Work out the finished part from the listing and answer in its coordinate system (mm). A direction names the side the tool comes from. Round coordinates to 2 decimals unless told otherwise and drop trailing zeros. Order: outer loops, then holes, each group sorted by start corner. A loop starts at its lowest first (then second) coordinate and runs counter-clockwise, first axis right, second up. Notation, with made-up numbers: (39, 29) -> (60, 29) arc R23 cw to (60, 58) -> close; hole circle Ø7 at (29.5, 17). An arc over 180 degrees is marked (long way). Use a Markdown table: item, result. Add a question column.
Item 1: Find the intervals of material crossed by L1, parallel to X at y = -52, z = 1.5; L2, parallel to Y at x = -55, z = 4.5 (3 decimals); L3, parallel to Z at x = 2.5, y = 0 (3 decimals), in increasing order. Write a range as [from, to].
Item 2: A cutting plane is placed at D-D, the plane x = -25. Determine the outline of the cut face in (y, z) (3 decimals), plus the area to 3 significant figures.
Item 3: A cutting plane is placed at C-C, the plane y = -50.5. Determine the outline of the cut face in (x, z).
Item 4: For a pull along X with two mould halves and no side action, classify faces 5 (the flat face through (-51, 38.1, 3)), 6 (the flat face through (-1, 1, 0)), 7 (the cylindrical face through (-72.38, 72.58, 3.13)) as +X half, -X half, draft (parallel to the pull), parting line (faces both ways), or undercut.
Item 5: A cutting plane is placed at B-B, the plane z = 3.5. Determine the outline of the cut face in (x, y) (3 decimals), plus the area to 3 significant figures.
Item 6: A cutting plane is placed at A-A, the plane y = 0. Determine the outline of the cut face in (x, z) (3 decimals), plus the area to 3 significant figures.
Item 7: A tool of negligible diameter and unlimited length cuts with its end or side. For faces 1 (the flat face through (51, -41.275, 3)), 2 (the flat face through (-31.75, -1, 25)), 3 (the flat face through (31.75, -1, 25)), 4 (the flat face through (0, 63.5, 19)), from which of +Z, -Z, +X, -X, +Y, -Y can it reach the whole face along a straight path? Write none if from no direction.
Item 8: Flat-ended cylindrical pins translate along their axes: P1, Ø4, axis at y = -54, z = 15.5, coming from the -X side; P2, Ø14.5, axis at y = 0, z = 15.875, coming from the +X side; P3, Ø3, axis at x = 26.5, z = 21.5, coming from the +Y side. Find the tip coordinate at first contact, or state that the pin passes through.
from build123d import *

# Parameters (mm, degrees)
F2_DEPTH = 6.35
F3_W     = 63.5
F3_H     = 127
F4_DEPTH = 25.4
F5_R     = 6.35
F6_DEPTH = 63.5
F7_W     = 12.7
F7_H     = 25.4
F8_DEPTH = 6.35


# Not quite as in the source:
# - the program builds the solid bodies; features that only make, move or delete a surface that nothing else refers to are left out


with BuildPart() as f2:
    # F0 (on Top) → F2 (new body)
    with BuildSketch(Plane.XY):
        with BuildLine():
            Line((63.5, 76.2), (-63.5, 76.2))
            ThreePointArc((-63.5, 76.2), (-72.4802561211, 72.4802561211), (-76.2, 63.5))
            Line((-76.2, 63.5), (-76.2, -63.5))
            ThreePointArc((-76.2, -63.5), (-72.4802561211, -72.4802561211), (-63.5, -76.2))
            Line((-63.5, -76.2), (63.5, -76.2))
            ThreePointArc((63.5, -76.2), (72.4802561211, -72.4802561211), (76.2, -63.5))
            Line((76.2, -63.5), (76.2, 63.5))
            ThreePointArc((76.2, 63.5), (72.4802561211, 72.4802561211), (63.5, 76.2))
        make_face()
        with BuildLine():
            ThreePointArc((-69.85, 57.15), (-66.1302561211, 66.1302561211), (-57.15, 69.85))
            Line((-57.15, 69.85), (-1.846e-07, 69.85))
            Line((-1.846e-07, 69.85), (57.15, 69.85))
            ThreePointArc((57.15, 69.85), (66.1302561211, 66.1302561211), (69.85, 57.15))
            Line((69.85, 57.15), (69.85, 0))
            Line((69.85, 0), (69.85, -57.15))
            ThreePointArc((69.85, -57.15), (66.1302561211, -66.1302561211), (57.15, -69.85))
            Line((57.15, -69.85), (0, -69.85))
            Line((0, -69.85), (-57.15, -69.85))
            ThreePointArc((-57.15, -69.85), (-66.1302561211, -66.1302561211), (-69.85, -57.15))
            Line((-69.85, -57.15), (-69.85, -1.807e-07))
            Line((-69.85, -1.807e-07), (-69.85, 57.15))
        make_face(mode=Mode.SUBTRACT)
        with BuildLine():
            ThreePointArc((69.85, 0), (49.3914086006, 49.3914087312), (-1.846e-07, 69.85))
            ThreePointArc((-1.846e-07, 69.85), (-49.3914087951, 49.3914085367), (-69.85, -1.807e-07))
            ThreePointArc((-69.85, -1.807e-07), (-49.391408602, -49.3914087298), (0, -69.85))
            ThreePointArc((0, -69.85), (49.3914086659, -49.3914086659), (69.85, 0))
        make_face()
        with BuildLine():
            Line((57.15, 69.85), (-1.846e-07, 69.85))
            ThreePointArc((-1.846e-07, 69.85), (49.3914086006, 49.3914087312), (69.85, 0))
            Line((69.85, 0), (69.85, 57.15))
            ThreePointArc((69.85, 57.15), (66.1302561211, 66.1302561211), (57.15, 69.85))
        make_face()
        with BuildLine():
            Line((-1.846e-07, 69.85), (-57.15, 69.85))
            ThreePointArc((-57.15, 69.85), (-66.1302561211, 66.1302561211), (-69.85, 57.15))
            Line((-69.85, 57.15), (-69.85, -1.807e-07))
            ThreePointArc((-69.85, -1.807e-07), (-49.3914087951, 49.3914085367), (-1.846e-07, 69.85))
        make_face()
        with BuildLine():
            Line((69.85, -57.15), (69.85, 0))
            ThreePointArc((69.85, 0), (49.3914086659, -49.3914086659), (0, -69.85))
            Line((0, -69.85), (57.15, -69.85))
            ThreePointArc((57.15, -69.85), (66.1302561211, -66.1302561211), (69.85, -57.15))
        make_face()
        with BuildLine():
            ThreePointArc((0, -69.85), (-49.391408602, -49.3914087298), (-69.85, -1.807e-07))
            Line((-69.85, -1.807e-07), (-69.85, -57.15))
            ThreePointArc((-69.85, -57.15), (-66.1302561211, -66.1302561211), (-57.15, -69.85))
            Line((-57.15, -69.85), (0, -69.85))
        make_face()
    extrude(amount=F2_DEPTH)

    # F3 (on face) → F4 (join)
    with BuildSketch(Plane.XY.offset(6.35)):
        Rectangle(F3_W, F3_H)
    extrude(amount=F4_DEPTH)

    # F5 (on face) → F6 (cut)
    with BuildSketch(Plane.YZ.offset(31.75)):
        with Locations((0, 15.875)):
            Circle(F5_R)
    extrude(amount=-F6_DEPTH, mode=Mode.SUBTRACT)

    # F7 (on face) → F8 (cut)
    with BuildSketch(Plane.XY.offset(6.35)):
        with Locations((50.8, 25.4)):
            Rectangle(F7_W, F7_H)
        with Locations((-50.8, 25.4)):
            Rectangle(F7_W, F7_H)
        with Locations((-50.8, -53.975)):
            Rectangle(F7_W, F7_H)
        with Locations((50.8, -53.975)):
            Rectangle(F7_W, F7_H)
    extrude(amount=-F8_DEPTH, mode=Mode.SUBTRACT)


solid = f2.part
Reported:
| question | item | result |
|---|---|---|
| 1 | L1 | [-76.2, -57.15], [-44.45, 44.45], [57.15, 76.2] |
| 1 | L2 | [-76.2, -66.675], [-41.275, 12.7], [38.1, 76.2] |
| 1 | L3 | [0, 9.525], [22.225, 31.75] |
| 2 | outline | (-76.2, 0) -> (76.2, 0) -> (76.2, 6.35) -> (63.5, 6.35) -> (63.5, 31.75) -> (-63.5, 31.75) -> (-63.5, 6.35) -> (-76.2, 6.35) -> close; hole circle Ø12.7 at (0, 15.875) |
| 2 | area | 4,070 mm² |
| 3 | outline | (-76.2, 0) -> (-57.15, 0) -> (-57.15, 6.35) -> (-76.2, 6.35) -> close; (-44.45, 0) -> (44.45, 0) -> (44.45, 6.35) -> (31.75, 6.35) -> (31.75, 31.75) -> (-31.75, 31.75) -> (-31.75, 6.35) -> (-44.45, 6.35) -> close; (57.15, 0) -> (76.2, 0) -> (76.2, 6.35) -> (57.15, 6.35) -> close |
| 4 | face 5 | undercut |
| 4 | face 6 | draft |
| 4 | face 7 | -X half |
| 5 | outline | (-76.2, -63.5) arc R12.7 ccw to (-63.5, -76.2) -> (63.5, -76.2) arc R12.7 ccw to (76.2, -63.5) -> (76.2, 63.5) arc R12.7 ccw to (63.5, 76.2) -> (-63.5, 76.2) arc R12.7 ccw to (-76.2, 63.5) -> close; hole (-57.15, -66.675) -> (-44.45, -66.675) -> (-44.45, -41.275) -> (-57.15, -41.275) -> close; hole (-57.15, 12.7) -> (-44.45, 12.7) -> (-44.45, 38.1) -> (-57.15, 38.1) -> close; hole (44.45, -66.675) -> (57.15, -66.675) -> (57.15, -41.275) -> (44.45, -41.275) -> close; hole (44.45, 12.7) -> (57.15, 12.7) -> (57.15, 38.1) -> (44.45, 38.1) -> close |
| 5 | area | 21,800 mm² |
| 6 | outline | (-76.2, 0) -> (76.2, 0) -> (76.2, 6.35) -> (31.75, 6.35) -> (31.75, 9.525) -> (-31.75, 9.525) -> (-31.75, 6.35) -> (-76.2, 6.35) -> close; (-31.75, 22.225) -> (31.75, 22.225) -> (31.75, 31.75) -> (-31.75, 31.75) -> close |
| 6 | area | 1,770 mm² |
| 7 | face 1 | +Z, -Z |
| 7 | face 2 | +Z, -X, +Y, -Y |
| 7 | face 3 | +Z, +X, +Y, -Y |
| 7 | face 4 | +Z, +X, -X, +Y |
| 8 | P1 | x = -31.75 |
| 8 | P2 | x = 31.75 |
| 8 | P3 | y = 63.5 |
